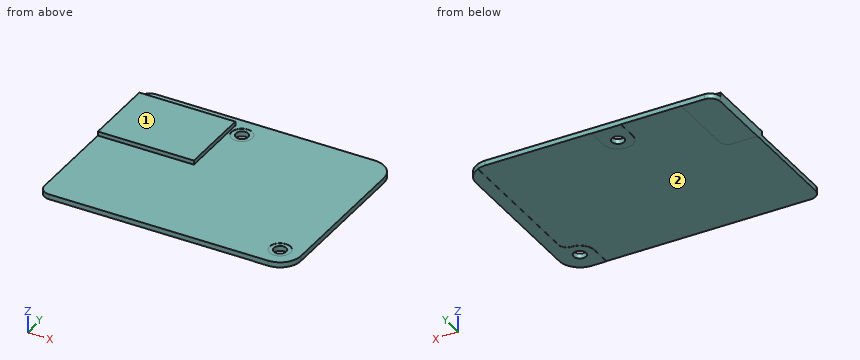
Autodesk Inventor part; units mm, degrees
ref_plane "YZ Plane" through (0, 0, 0) normal (1, 0, 0) x (0, 1, 0)
ref_plane "XZ Plane" through (0, 0, 0) normal (0, 1, 0) x (-1, 0, 0)
ref_plane "XY Plane" through (0, 0, 0) normal (0, 0, 1) x (1, 0, 0)
sketch "Sketch1" plane through (0, 0, 0) normal (0, 0, 1) x (1, 0, 0)
  line L0 (10.25, 20.1716) -> (10.25, 23.6716)
  line L1 (-1.25, 23.6716) -> (10.25, 23.6716)
  arc A0 (0.75, 23.3284) -> (-1.25, 23.6716) centre (-1.25, 17.6716) ccw
  line L2 (0.75, 23.3284) -> (0.75, -11.8284)
  arc A1 (-1.25, -13.8284) -> (0.75, -11.8284) centre (-1.25, -11.8284) ccw
  arc A2 (-1.25, -13.8284) -> (-4.75, -17.3284) centre (-1.25, -17.3284) ccw
  line L3 (-4.75, -17.3284) -> (-4.75, -23.3284)
  line L4 (10.25, -23.3284) -> (-4.75, -23.3284)
  line L5 (10.25, -23.3284) -> (10.25, -19.8284)
  line L6 (10.25, -19.8284) -> (6.75, -19.8284)
  line L7 (6.75, -19.8284) -> (6.75, 8.1716)
  line L8 (6.75, 8.1716) -> (16.75, 8.1716)
  line L9 (16.75, 17.1716) -> (16.75, 8.1716)
  line L10 (16.75, 17.1716) -> (13.25, 17.1716)
  arc A3 (10.25, 20.1716) -> (13.25, 17.1716) centre (13.25, 20.1716) ccw
  circle A4 centre (-1.25, -17.3284) radius 1.5
  line L11 (-57.25, 4.6716) -> (-57.25, 20.1716)
  line L12 (-57.25, 4.6716) -> (-50.25, 4.6716)
  arc A5 (-50.25, 4.6716) -> (-48.25, 6.6716) centre (-50.25, 6.6716) ccw
  line L13 (-48.25, 6.6716) -> (-48.25, 23.6716)
  line L14 (-53.75, 23.6716) -> (-48.25, 23.6716)
  arc A6 (-53.75, 23.6716) -> (-57.25, 20.1716) centre (-53.75, 20.1716) ccw
  line L15 (-26.75, 17.6716) -> (-26.75, 23.6716)
  line L16 (-33.75, 23.6716) -> (-26.75, 23.6716)
  line L17 (-33.75, 23.6716) -> (-33.75, 17.6716)
  arc A7 (-33.75, 17.6716) -> (-26.75, 17.6716) centre (-30.25, 17.6716) ccw
  circle A8 centre (-30.25, 17.6716) radius 1.5
  line L18 (-50.25, 4.6716) -> (-57.25, 4.6716)
  line L19 (-57.25, -19.8284) -> (-57.25, 4.6716)
  arc A9 (-57.25, -19.8284) -> (-53.75, -23.3284) centre (-53.75, -19.8284) ccw
  line L20 (-4.75, -23.3284) -> (-53.75, -23.3284)
  line L21 (-4.75, -23.3284) -> (-4.75, -17.3284)
  arc A10 (-1.25, -13.8284) -> (-4.75, -17.3284) centre (-1.25, -17.3284) ccw
  arc A11 (-1.25, -13.8284) -> (0.75, -11.8284) centre (-1.25, -11.8284) ccw
  line L22 (0.75, -11.8284) -> (0.75, 23.3284)
  arc A12 (0.75, 23.3284) -> (-1.25, 23.6716) centre (-1.25, 17.6716) ccw
  line L23 (-26.75, 23.6716) -> (-1.25, 23.6716)
  line L24 (-26.75, 23.6716) -> (-26.75, 17.6716)
  arc A13 (-33.75, 17.6716) -> (-26.75, 17.6716) centre (-30.25, 17.6716) ccw
  line L25 (-33.75, 17.6716) -> (-33.75, 23.6716)
  line L26 (-48.25, 23.6716) -> (-33.75, 23.6716)
  line L27 (-48.25, 23.6716) -> (-48.25, 6.6716)
  arc A14 (-50.25, 4.6716) -> (-48.25, 6.6716) centre (-50.25, 6.6716) ccw
  line L28 (-1.25, -17.3284) -> (-53.75, -17.3284) construction
  line L29 (-53.75, -17.3284) -> (-53.75, 20.1716) construction
  line L30 (-53.75, 20.1716) -> (-1.25, 20.1716) construction
  line L31 (-1.25, 20.1716) -> (-1.25, -17.3284) construction
  arc A15 (-1.25, -22.3284) -> (3.75, -17.3284) centre (-1.25, -17.3284) ccw
  line L32 (-1.25, -22.3284) -> (-4.75, -22.3284)
  line L33 (3.75, -17.3284) -> (3.75, 17.6716)
  arc A16 (3.75, 17.6716) -> (0.75, 22.2541) centre (-1.25, 17.6716) ccw
  line L34 (-56.25, 4.6716) -> (-56.25, 20.1716)
  line L35 (-48.25, 22.6716) -> (-53.75, 22.6716)
  arc A17 (-53.75, 22.6716) -> (-56.25, 20.1716) centre (-53.75, 20.1716) ccw
  line L36 (-26.75, 22.6716) -> (-33.75, 22.6716)
  point P0 (0, 0)
  dimension "d0" = 5
  dimension "d1" = 2.5
extrude "Extrusion1" add sketch "Sketch1" along normal blind 0.05 contours A16 L33 A15 L32 L3 A2 A1 L2 | L15 A7 L17 L36 | L13 A5 L12 L34 A17 L35
sketch "Sketch2" plane through (0, 0, 0.05) normal (0, 0, 1) x (1, 0, 0)
  arc A0 (3.75, 17.6716) -> (0.75, 22.2541) centre (-1.25, 17.6716) ccw
  line L0 (0.75, 22.2541) -> (0.75, -11.8284)
  arc A1 (-1.25, -13.8284) -> (0.75, -11.8284) centre (-1.25, -11.8284) ccw
  arc A2 (-1.25, -13.8284) -> (-4.75, -17.3284) centre (-1.25, -17.3284) ccw
  line L1 (-4.75, -17.3284) -> (-4.75, -22.3284)
  line L2 (-4.75, -22.3284) -> (-1.25, -22.3284)
  arc A3 (-1.25, -22.3284) -> (3.75, -17.3284) centre (-1.25, -17.3284) ccw
  line L3 (3.75, -17.3284) -> (3.75, 17.6716)
  circle A4 centre (-1.25, -17.3284) radius 1.5
  line L4 (-56.25, 20.1716) -> (-56.25, 4.6716)
  line L5 (-56.25, 4.6716) -> (-50.25, 4.6716)
  arc A5 (-50.25, 4.6716) -> (-48.25, 6.6716) centre (-50.25, 6.6716) ccw
  line L6 (-48.25, 6.6716) -> (-48.25, 22.6716)
  line L7 (-48.25, 22.6716) -> (-53.75, 22.6716)
  arc A6 (-53.75, 22.6716) -> (-56.25, 20.1716) centre (-53.75, 20.1716) ccw
  arc A7 (0.75, 22.2541) -> (-1.25, 22.6716) centre (-1.25, 17.6716) ccw
  line L8 (-1.25, 22.6716) -> (-48.25, 22.6716)
  arc A8 (-57.1041, -20.8284) -> (-53.75, -23.3284) centre (-53.75, -19.8284) ccw
  arc A9 (-56.25, -19.8284) -> (-53.75, -22.3284) centre (-53.75, -19.8284) ccw
  line L9 (-4.75, -22.3284) -> (-53.75, -22.3284)
  line L10 (-56.25, -19.8284) -> (-56.25, 4.6716)
  circle A10 centre (-30.25, 17.6716) radius 1.5
  point P0 (0, 0)
extrude "Extrusion2" add sketch "Sketch2" along normal blind 1.2
sketch "Sketch3" plane through (0, 0, 1.25) normal (0, 0, 1) x (1, 0, 0)
  arc A0 (-56.25, -19.8284) -> (-53.75, -22.3284) centre (-53.75, -19.8284) ccw
  line L0 (-53.75, -22.3284) -> (-1.25, -22.3284)
  arc A1 (-1.25, -22.3284) -> (3.75, -17.3284) centre (-1.25, -17.3284) ccw
  line L1 (3.75, -17.3284) -> (3.75, 17.6716)
  arc A2 (3.75, 17.6716) -> (-1.25, 22.6716) centre (-1.25, 17.6716) ccw
  line L2 (-1.25, 22.6716) -> (-53.75, 22.6716)
  arc A3 (-53.75, 22.6716) -> (-56.25, 20.1716) centre (-53.75, 20.1716) ccw
  line L3 (-56.25, 20.1716) -> (-56.25, -19.8284)
  circle A4 centre (-1.25, -17.3284) radius 1.5
  circle A5 centre (-30.25, 17.6716) radius 1.5
  circle A6 centre (-1.25, -17.3284) radius 1.5
  circle A7 centre (-1.25, -17.3284) radius 2.5
  circle A8 centre (-30.25, 17.6716) radius 2.5
  point P0 (0, 0)
  dimension "d6" = 5
  dimension "d7" = 5
extrude "Extrusion3" cut sketch "Sketch3" against normal blind 0.05 contours A4 | A5 | A7 | A8
sketch "Sketch4" plane through (0, 0, 1.25) normal (0, 0, 1) x (1, 0, 0)
  line L0 (-56.25, 20.1716) -> (-56.25, -19.8284)
  line L1 (-56.25, 20.1716) -> (-33.25, 20.1716)
  line L2 (-33.25, 20.1716) -> (-33.25, 2.6716)
  line L3 (-33.25, 2.6716) -> (-56.25, 2.6716)
  line L4 (-56.25, 2.6716) -> (-56.25, 20.1716)
  point P0 (0, 0)
  point P1 (-56.25, 2.6716)
  dimension "d10" = 17.5
  dimension "d11" = 23
extrude "Extrusion4" add sketch "Sketch4" along normal blind 1
properties material "Phenolic Resin"
Geometry check sheet. Reference: the model listing, model coordinates, mm. Face numbers are marked on the shaded views. Give positions to 0.01 mm unless a question says otherwise; leave off trailing zeros. Write each loop counter-clockwise with the first axis right and the second up, starting at its lowest first coordinate (ties: lowest second). Pieces come first, ordered by that corner, then holes. Notation, with made-up numbers: (-16.75, 79) -> (8.25, 79) arc R23 cw to (8.25, 93) -> close; hole circle Ø1 at (-24, -38.75). An arc over 180 degrees is marked (long way). Use one line per item in the form item = value.
Item 1: Depth check by flat-ended pin: pin 1 Ø4.5 at (x, y) = (-1.25, -17.33) entering from -Z; pin 2 Ø10 at (x, y) = (-17, 14.5) entering from +Z; pin 3 Ø2.5 at (x, y) = (-30.25, 17.67) entering from +Z. Enter the tip coordinate at first touch or a pass-through.
Results list:
pin_1 = 0
pin_2 = 1.25
pin_3 = through
Item 2: Mould release check, pull along X, two halves, no side actions. Record for the marked faces 1 and 2: released by +X, released by -X, zero draft, split by the parting line, or undercut.
Results list:
face_1 = zero draft
face_2 = undercut
Item 3: Sectioned sample at B-B on y = 0. Enter the section's corners in (x, z), plus the area to 4 significant figures.
Results list:
outline = (-56.25, 0.05) -> (0.75, 0.05) -> (0.75, 0) -> (3.75, 0) -> (3.75, 1.25) -> (-56.25, 1.25) -> close
area = 72.15 mm2
Item 4: Sectioned sample at A-A on x = -30.25. Enter the section's corners in (y, z).
Results list:
outline = (-22.33, 0.05) -> (14.17, 0.05) -> (14.17, 0) -> (16.17, 0) -> (16.17, 1.2) -> (15.17, 1.2) -> (15.17, 1.25) -> (-22.33, 1.25) -> close; (19.17, 0) -> (22.67, 0) -> (22.67, 1.25) -> (20.17, 1.25) -> (20.17, 1.2) -> (19.17, 1.2) -> close
Item 5: Scan lines: line 1 (Y direction, x = -1.25, z = 0.7); line 2 (Z direction, x = -28, y = 10); line 3 (X direction, y = -16, z = 0.25). Record each from-to range of solid material in increasing order.
Results list:
line_1 = -22.33 to -18.83, -15.83 to 22.67
line_2 = 0.05 to 1.25
line_3 = -56.25 to -1.95, -0.55 to 3.75
